Verification items for this drawing (mm, ordinates from the low corner). Give positions to 0.01 mm unless a question says otherwise; leave off trailing zeros. Write each loop counter-clockwise with the first axis right and the second up, starting at its lowest first coordinate (ties: lowest second). Pieces come first, ordered by that corner, then holes. Notation, with made-up numbers: (-29.5, 68) -> (-10.5, 68) arc R21 ccw to (-10.5, 78) -> close; hole circle Ø5 at (28.25, -3.5). An arc over 180 degrees is marked (long way). Use one line per item in the form item = value. Start each with the question number.
(1) Section check D-D, the plane y = 2. Record the cut outline in (x, z).
(2) Scan lines: L1, parallel to Y at x = 4.5, z = 1.05 (1 decimal); L2, parallel to Y at x = 2.25, z = 0.25 (1 decimal); L3, parallel to X at y = 8, z = 0.6. Record each from-to range of solid material in increasing order.
(3) Release check for a two-part mould opening along Y. For the marked faces 1, 2, 3 and 4 record: pulls with the +Y half, pulls with the -Y half, needs draft (parallel to the pull), parting line crosses it, or undercut.
(4) Depth check by flat-ended pin: pin 1 Ø1 at (x, z) = (7, 1.5) entering from -Y. Enter the tip coordinate at first touch or a pass-through.
(5) Section check B-B, the plane y = 10.75. Record the cut outline in (x, z) (1 decimal).
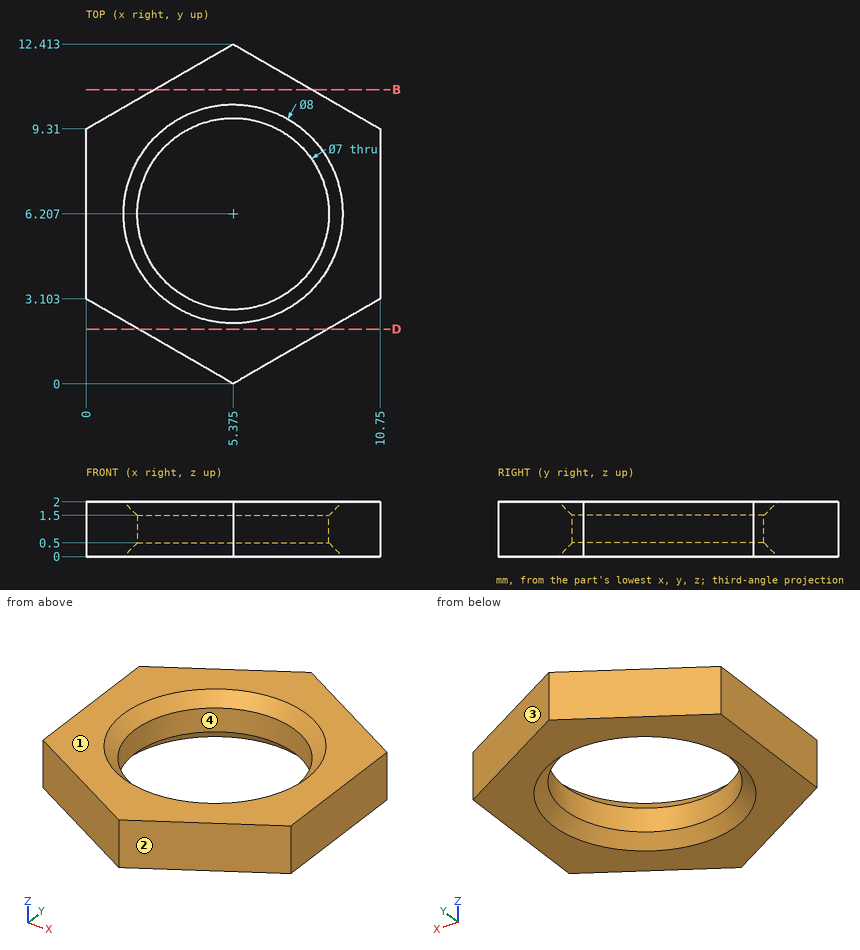
Completed:
q1.outline = (1.91, 0) -> (8.84, 0) -> (8.84, 2) -> (1.91, 2) -> close
q2.L1 = 0.5 to 2.8, 9.6 to 11.9
q2.L2 = 1.8 to 4.1, 8.3 to 10.6
q2.L3 = 0 to 2.37, 8.38 to 10.75
q3.face_1 = needs draft
q3.face_2 = pulls with the -Y half
q3.face_3 = pulls with the +Y half
q3.face_4 = undercut
q4.pin_1 = 0.65
q5.outline = (2.5, 0) -> (8.3, 0) -> (8.3, 2) -> (2.5, 2) -> close
